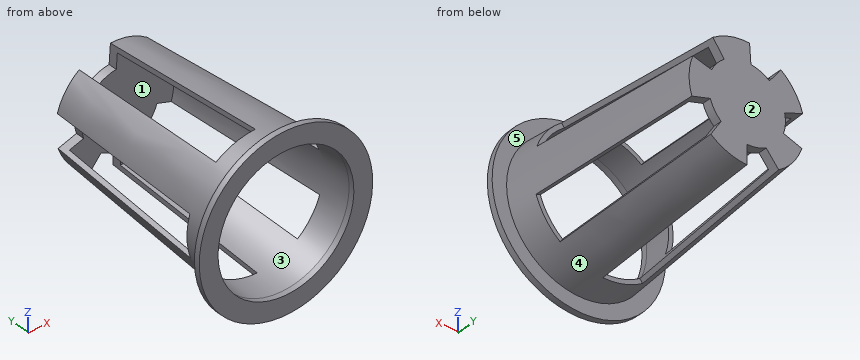
from build123d import *

# Parameters (mm, degrees)
SKETCH6_R           = 20
SKETCH4_R           = 25
SKETCH8_R           = 18.5
SKETCH7_R           = 23.5
SKETCH9_R           = 30
BOSS_EXTRUDE1_DEPTH = 2
SKETCH10_R          = 23.5
CUT_EXTRUDE2_DEPTH  = 2
CUT_EXTRUDE4_DEPTH  = 60


with BuildPart() as part:
    # Sketch6 → Loft1 section 0
    with BuildSketch(Plane(origin=(0, 70, 0), x_dir=(1, 0, 0), z_dir=(0, 1, 0))):
        Circle(SKETCH6_R)
    # Sketch4 → Loft1 section 1
    with BuildSketch(Plane(origin=(0, 0, 0), x_dir=(1, 0, 0), z_dir=(0, 1, 0))):
        Circle(SKETCH4_R)
    loft()

    # Sketch8 → Cut-Loft2 section 0
    with BuildSketch(Plane(origin=(0, 67, 0), x_dir=(1, 0, 0), z_dir=(0, 1, 0))):
        Circle(SKETCH8_R)
    # Sketch7 → Cut-Loft2 section 1
    with BuildSketch(Plane.XZ):
        Circle(SKETCH7_R)
    loft(mode=Mode.SUBTRACT)

    # Sketch9 → Boss-Extrude1 (add)
    with BuildSketch(Plane(origin=(0, 0, 0), x_dir=(1, 0, 0), z_dir=(0, 1, 0))):
        with Locations(Location((0, 0, 0), (0, 0, 270))):
            Circle(SKETCH9_R)
    extrude(amount=-BOSS_EXTRUDE1_DEPTH)

    # Sketch10 → Cut-Extrude2 (cut)
    with BuildSketch(Plane.XZ.offset(2)):
        with Locations(Location((0, 0, 0), (0, 0, 270))):
            Circle(SKETCH10_R)
    extrude(amount=-CUT_EXTRUDE2_DEPTH, mode=Mode.SUBTRACT)

    # Sketch11 → Cut-Extrude4 (cut)
    with BuildSketch(Plane(origin=(0, 70, 0), x_dir=(1, 0, 0), z_dir=(0, 1, 0))):
        with BuildLine():
            Line((0, 13.334004414), (0, 25))
            ThreePointArc((0, 25), (-7.452245669, 23.86344557), (-14.226900712, 20.557122759))
            Line((-14.226900712, 20.557122759), (-6.667002207, 11.547586557))
            ThreePointArc((-6.667002207, 11.547586557), (-3.45109429, 12.879659232), (0, 13.334004414))
        make_face()
        with BuildLine():
            Line((12.681391787, 4.120433967), (23.776412907, 7.725424859))
            ThreePointArc((23.776412907, 7.725424859), (20.392614853, 14.46171703), (15.154631459, 19.883086917))
            Line((15.154631459, 19.883086917), (8.922190459, 9.909096384))
            ThreePointArc((8.922190459, 9.909096384), (11.182837055, 7.262219297), (12.681391787, 4.120433967))
        make_face()
        with BuildLine():
            Line((7.837531149, -10.787436174), (14.694631307, -20.225424859))
            ThreePointArc((14.694631307, -20.225424859), (20.055574767, -14.92561291), (23.59297804, -8.268699244))
            Line((23.59297804, -8.268699244), (12.181219165, -5.423428194))
            ThreePointArc((12.181219165, -5.423428194), (10.362467681, -8.391360872), (7.837531149, -10.787436174))
        make_face()
        with BuildLine():
            Line((-7.837531149, -10.787436174), (-14.694631307, -20.225424859))
            ThreePointArc((-14.694631307, -20.225424859), (-7.997587983, -23.686253111), (-0.573369135, -24.993424092))
            Line((-0.573369135, -24.993424092), (-1.393782991, -13.260959343))
            ThreePointArc((-1.393782991, -13.260959343), (-4.778479821, -12.448365528), (-7.837531149, -10.787436174))
        make_face()
        with BuildLine():
            Line((-12.681391787, 4.120433967), (-23.776412907, 7.725424859))
            ThreePointArc((-23.776412907, 7.725424859), (-24.998355969, 0.286703421), (-23.947339654, -7.17808634))
            Line((-23.947339654, -7.17808634), (-13.042624426, -2.772295403))
            ThreePointArc((-13.042624426, -2.772295403), (-13.315730625, 0.697847872), (-12.681391787, 4.120433967))
        make_face()
    extrude(amount=-CUT_EXTRUDE4_DEPTH, mode=Mode.SUBTRACT)


solid = part.part
Verification items for the finished model (mm, model axes). Face numbers are marked on the shaded views. A direction names the side the tool comes from. Coordinates: 2 decimals unless noted, no trailing zeros. Order: outer loops, then holes, each group sorted by start corner. A loop starts at its lowest first (then second) coordinate and runs counter-clockwise, first axis right, second up.
Item 1: Material ranges on L1, parallel to X at y = -1.4, z = 0; L2, parallel to Y at x = 4.5, z = 13; L3, parallel to Z at x = 8, y = 11, recorded low to high.
Filled in:
L1: x = -30 to -23.5, 23.5 to 30
L2: y = 67 to 70
L3: z = -22.85 to -21.22, 21.22 to 22.85
Item 2: Section check A-A, the plane y = 13. Enter the section's corners in (x, z).
Filled in:
outline: (-23.08, 6.83) - (-21.65, 6.25) arc R22.53 cw to (-13.24, 18.23) - (-14.15, 19.47) arc R24.07 ccw to start; (-22.89, -7.44) arc R24.07 ccw to (-13.63, -19.84) - (-12.63, -18.66) arc R22.53 cw to (-21.43, -6.96) - close; (-0.75, 22.52) arc R22.53 cw to (13.24, 18.23) - (14.15, 19.47) arc R24.07 ccw to (-0.64, 24.06) - close; (0, -24.07) arc R24.07 ccw to (14.66, -19.09) - (13.84, -17.78) arc R22.53 cw to (0, -22.53) - close; (21.18, 7.67) arc R22.53 cw to (21.43, -6.96) - (22.89, -7.44) arc R24.07 ccw to (22.69, 8.04) - close
Item 3: Access from +Z, -Z, +X, -X, +Y, -Y to the whole of each face (thin tool, end or side, straight path). Record for the marked faces 1 and 2.
Filled in:
face 1: -Y
face 2: +Z, -Z, +X, -X, +Y
Item 4: Depth check by flat-ended pin: pin 1 (4.5 mm diameter, centred on x = -7, z = 21.5, fed in from +Y); pin 2 (1.5 mm diameter, centred on y = 51, z = -9, fed in from -X); pin 3 (10 mm diameter, centred on y = 7.5, z = 19.5, fed in from +X). Enter the tip coordinate at first touch or a pass-through.
Filled in:
pin 1: stops at y = 10
pin 2: stops at x = -19.7
pin 3: stops at x = 19.73
Item 5: Release check for a two-part mould opening along Z. For the marked faces 3, 4 and 5 record: +Z half, -Z half, draft (parallel to the pull), parting line (faces both ways), or undercut.
Filled in:
face 3: undercut
face 4: parting line
face 5: draft
Item 6: Section check B-B, the plane y = 60.5. Enter the section's corners in (x, z), then the cut area to 3 significant figures.
Filled in:
outline: (-19.92, 5.55) - (-18.34, 4.91) arc R18.99 cw to (-11.16, 15.36) - (-12.15, 16.73) arc R20.68 ccw to start; (-19.67, -6.39) arc R20.68 ccw to (-11.43, -17.23) - (-10.34, -15.92) arc R18.99 cw to (-18.06, -5.87) - close; (-1, 18.96) arc R18.99 cw to (11.16, 15.36) - (12.15, 16.73) arc R20.68 ccw to (-0.88, 20.66) - close; (0, -20.68) arc R20.68 ccw to (12.85, -16.2) - (11.95, -14.75) arc R18.99 cw to (0, -18.99) - close; (17.72, 6.81) arc R18.99 cw to (18.06, -5.87) - (19.67, -6.39) arc R20.68 ccw to (19.38, 7.22) - close
area: 113 mm2
